from build123d import *

# Parameters (mm, degrees)
F1_DEPTH = 12.7
F2_R     = 23.876
F3_DEPTH = 12.701
F4_R     = 3.175
F5_DEPTH = 25.4


with BuildPart() as f1:
    # F0 (on Right) → F1 (new body)
    with BuildSketch(Plane.YZ):
        Polygon((12.7, 88.9), (0, 88.9), (-12.7, 88.9), (-31.75, 69.85), (-31.75, -88.9), (0, -88.9), (31.75, -88.9), (31.75, 69.85), align=None)
    extrude(amount=F1_DEPTH)

    # F2 (on Right) → F3 (cut, through all)
    with BuildSketch(Plane.YZ):
        with Locations((0, 50.8)):
            Circle(F2_R)
    extrude(amount=F3_DEPTH, mode=Mode.SUBTRACT)

    # F4 (on face) → F5 (cut)
    with BuildSketch(Plane(origin=(0, 0, -88.9), x_dir=(1, 0, 0), z_dir=(0, 0, -1))):
        with Locations((6.35, 19.05)):
            Circle(F4_R)
        with Locations((6.35, -19.05)):
            Circle(F4_R)
    extrude(amount=-F5_DEPTH, mode=Mode.SUBTRACT)


solid = f1.part
Input: part model. Units: mm. Frame: model coordinates. A direction names the side the tool comes from. Give positions to 0.01 mm unless a question says otherwise; leave off trailing zeros. Write each loop counter-clockwise with the first axis right and the second up, starting at its lowest first coordinate (ties: lowest second). Pieces come first, ordered by that corner, then holes. Notation, with made-up numbers: M 48.5,69.25 L 88.5,69.25 A28 cw 88.5,101.25 Z; hole C 60.5,64.5 d8. An arc over 180 degrees is marked long. Write item = value, one per line. Start each with the question number.
1) Draft query along X for faces 1 (the cylindrical face through (5.66, -15.95, -76.38)), 2 (the cylindrical face through (3.18, 18.91, -76.38)), 3 (the flat face through (12.7, 0, -19)), 4 (the flat face through (6, 31.75, -11)). Return one class per face: +X half, -X half, draft (parallel to the pull), parting line (faces both ways), or undercut.
2) Material intervals for line 1 along Y through (x, z) = (6.35, -71.25) (3 decimals); line 2 along Z through (x, y) = (9.5, 0); line 3 along X through (y, z) = (19.05, -74.75) (3 decimals), sorted ascending. Write a range as [from, to].
3) Cut plane B-B on z = 50.8. Return the cut outline in (x, y), then the cut area to 3 significant figures.
4) Cut plane C-C on x = 6.35. Return the cut outline in (y, z) (3 decimals).
5) Cut plane A-A on y = 0. Return the cut outline in (x, z).
6) Cut plane D-D on z = -67.5. Return the cut outline in (x, y) (3 decimals).
7) First-contact query: pin 1 Ø5.5 at (x, y) = (6.35, -19.05) entering from -Z. Flat tip, straight axial feed; report the tip coordinate or a pass-through.
8) Reachability of faces 5 (the flat face through (6, -19, -63.5)), 6 (the flat face through (6.3, 22.4, 79.2)) from +Z, -Z, +X, -X, +Y, -Y: full face, straight path, thin tool, end or side. Return the list, or none.
Solved:
q1.face_1 = undercut
q1.face_2 = undercut
q1.face_3 = +X half
q1.face_4 = draft
q2.line_1 = [-31.75, -22.225], [-15.875, 15.875], [22.225, 31.75]
q2.line_2 = [-88.9, 26.92], [74.68, 88.9]
q2.line_3 = [0, 3.175], [9.525, 12.7]
q3.outline = M 0,-31.75 L 12.7,-31.75 L 12.7,-23.88 L 0,-23.88 Z; M 0,23.88 L 12.7,23.88 L 12.7,31.75 L 0,31.75 Z
q3.area = 200 mm2
q4.outline = M -31.75,-88.9 L -22.225,-88.9 L -22.225,-63.5 L -15.875,-63.5 L -15.875,-88.9 L 15.875,-88.9 L 15.875,-63.5 L 22.225,-63.5 L 22.225,-88.9 L 31.75,-88.9 L 31.75,69.85 L 12.7,88.9 L -12.7,88.9 L -31.75,69.85 Z; hole C 0,50.8 d47.752
q5.outline = M 0,-88.9 L 12.7,-88.9 L 12.7,26.92 L 0,26.92 Z; M 0,74.68 L 12.7,74.68 L 12.7,88.9 L 0,88.9 Z
q6.outline = M 0,-31.75 L 12.7,-31.75 L 12.7,31.75 L 0,31.75 Z; hole C 6.35,-19.05 d6.35; hole C 6.35,19.05 d6.35
q7.pin_1 = -63.5
q8.face_5 = -Z
q8.face_6 = +Z, +X, -X, +Y
